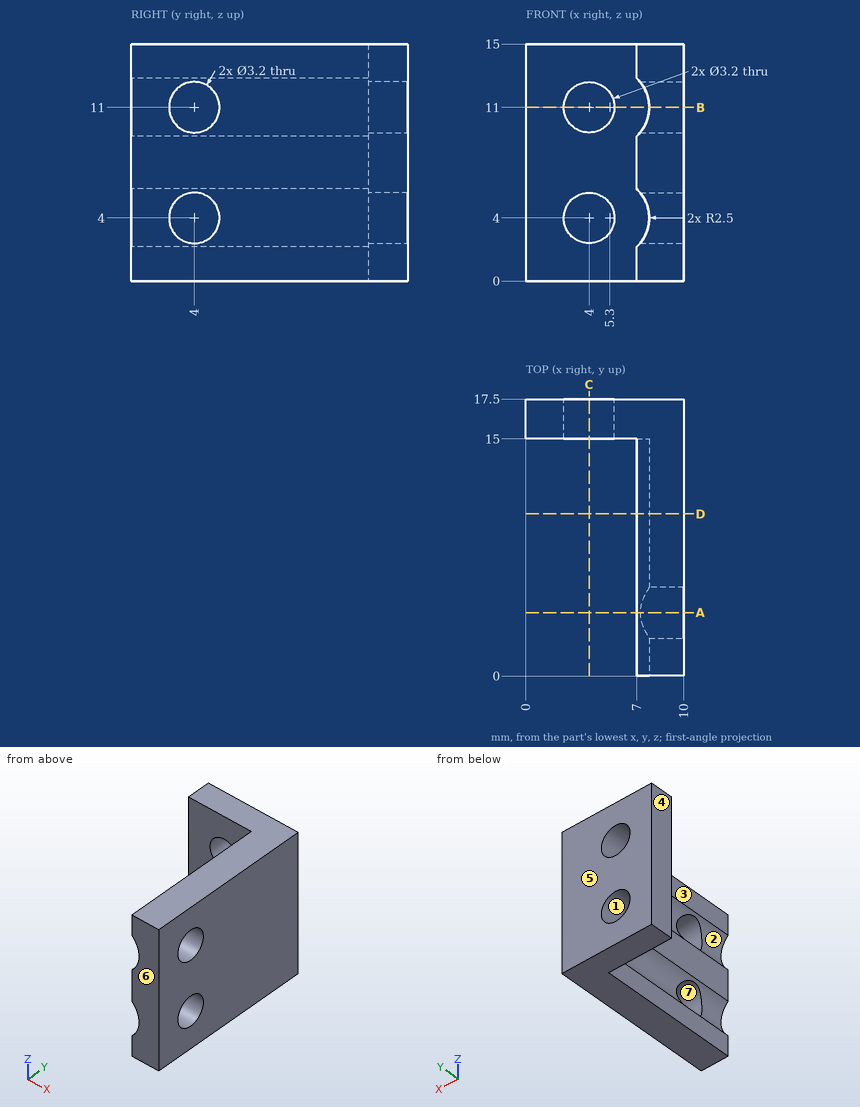
Part print with two shaded views. Sizes in mm from the minimum x, y, z corner. A direction names the side the tool comes from. Round coordinates to 2 decimals unless told otherwise and drop trailing zeros. Loops run counter-clockwise (first coordinate to the right, second up) from the corner with the lowest first, then second, coordinate; pieces in that order, holes last.
Item 1: Saw through at D-D (y = 10.25). List the corners of the cut face in (x, z).
Item 2: Saw through at C-C (x = 4). List the corners of the cut face in (y, z).
Item 3: Two-plate mould, pull along Y, no slides. Class the marked faces 4, 5, 6 and 7: released by +Y, released by -Y, zero draft, split by the parting line, or undercut.
Item 4: Saw through at B-B (z = 11). List the corners of the cut face in (x, y), then the cut area to 3 significant figures.
Item 5: Drill centre lines: line 1 along Z through (x, y) = (8.4, 4); line 2 along Y through (x, z) = (8.65, 11); line 3 along X through (y, z) = (17, 4). Where is each one in solid material? Low to high.
Item 6: Which spindle directions (+Z, -Z, +X, -X, +Y, -Y) get a long thin tool onto all of the face, cutting with end or side? Do the marked faces 1, 2 and 3. Say none if no direction does.
Item 7: Saw through at A-A (y = 4). List the corners of the cut face in (x, z).
Item 8: Pin check, flat tips, straight feed: P1, Ø2.5, axis at y = 5, z = 13.5, coming from the -X side; P2, Ø4, axis at y = 4, z = 11, coming from the +X side. Stop position of each tip, or through.
Worked answers:
1. outline: (7, 0) - (10, 0) - (10, 15) - (7, 15) - (7, 12.83) arc R2.5 cw to (7, 9.17) - (7, 5.83) arc R2.5 cw to (7, 2.17) - close
2. outline: (15, 0) - (17.5, 0) - (17.5, 2.4) - (15, 2.4) - close; (15, 5.6) - (17.5, 5.6) - (17.5, 9.4) - (15, 9.4) - close; (15, 12.6) - (17.5, 12.6) - (17.5, 15) - (15, 15) - close
3. face 4: zero draft
3. face 5: released by +Y
3. face 6: released by -Y
3. face 7: undercut
4. outline: (0, 15) - (2.4, 15) - (2.4, 17.5) - (0, 17.5) - close; (5.6, 15) - (7.8, 15) - (7.8, 5.6) - (10, 5.6) - (10, 17.5) - (5.6, 17.5) - close; (7.8, 0) - (10, 0) - (10, 2.4) - (7.8, 2.4) - close
4. area: 43.0 mm2
5. line 1: z = 0 to 2.4, 5.6 to 9.4, 12.6 to 15
5. line 2: y = 0 to 2.4, 5.6 to 17.5
5. line 3: x = 0 to 2.4, 5.6 to 10
6. face 1: +Y, -Y
6. face 2: -X, -Y
6. face 3: +Z, -Z, -X, -Y
7. outline: (7, 0) - (10, 0) - (10, 2.4) - (7.22, 2.4) arc R2.5 cw to (7, 2.17) - close; (7, 5.83) arc R2.5 cw to (7.22, 5.6) - (10, 5.6) - (10, 9.4) - (7.22, 9.4) arc R2.5 cw to (7, 9.17) - close; (7, 12.83) arc R2.5 cw to (7.22, 12.6) - (10, 12.6) - (10, 15) - (7, 15) - close
8. P1: stops at x = 7
8. P2: stops at x = 10
